```python
from build123d import *

# Parameters (mm, degrees)
F0_R           = 55
F1_DEPTH       = 8
F3_D           = 4
F4_D           = 3.75
F4_CBORE_D     = 6.75
F4_CBORE_DEPTH = 3
F5_W           = 80.514036
F5_H           = 245.416
F5_W_2         = 74.904691
F6_DEPTH       = 25


with BuildPart() as f1:
    # F0 (on Top) → F1 (new body)
    with BuildSketch(Plane.XY):
        with BuildLine():
            Line((105, 90), (105, 105))
            Line((105, 105), (90, 105))
            add(Edge.make_bspline(
                [(-90, 105), (-90, 62.5), (0, 62.5), (90, 62.5), (90, 105)],
                knots=[3.141593, 3.141593, 3.141593, 4.712389, 4.712389, 6.283185, 6.283185, 6.283185], degree=2, weights=[1, 0.707107, 1, 0.707107, 1]))
            Line((-90, 105), (-105, 105))
            Line((-105, 105), (-105, 90))
            add(Edge.make_bspline(
                [(-105, -90), (-62.5, -90), (-62.5, 0), (-62.5, 90), (-105, 90)],
                knots=[3.141593, 3.141593, 3.141593, 4.712389, 4.712389, 6.283185, 6.283185, 6.283185], degree=2, weights=[1, 0.707107, 1, 0.707107, 1]))
            Line((-105, -90), (-105, -105))
            Line((-105, -105), (-90, -105))
            add(Edge.make_bspline(
                [(90, -105), (90, -62.5), (0, -62.5), (-90, -62.5), (-90, -105)],
                knots=[0, 0, 0, 1.570796, 1.570796, 3.141593, 3.141593, 3.141593], degree=2, weights=[1, 0.707107, 1, 0.707107, 1]))
            Line((90, -105), (105, -105))
            Line((105, -105), (105, -90))
            add(Edge.make_bspline(
                [(105, 90), (62.5, 90), (62.5, 0), (62.5, -90), (105, -90)],
                knots=[0, 0, 0, 1.570796, 1.570796, 3.141593, 3.141593, 3.141593], degree=2, weights=[1, 0.707107, 1, 0.707107, 1]))
        make_face()
        Circle(F0_R, mode=Mode.SUBTRACT)
    extrude(amount=F1_DEPTH)

    # F3 (through all)
    with Locations(Plane.XY.offset(8)):
        with Locations((-100, 100), (100, 100), (100, -100), (-100, -100)):
            Hole(F3_D / 2)

    # F4 (through all)
    with Locations(Plane.XY.offset(8)):
        with Locations((-50, 50), (-50, -50), (50, -50), (50, 50)):
            CounterBoreHole(F4_D / 2, F4_CBORE_D / 2, F4_CBORE_DEPTH)

    # F5 (on Top) → F6 (cut)
    with BuildSketch(Plane.XY):
        Rectangle(F5_W, F5_H)
        with Locations((77.709363, 0)):
            Rectangle(F5_W_2, F5_H)
    extrude(amount=F6_DEPTH, mode=Mode.SUBTRACT)


solid = f1.part
```
Geometry check sheet. Reference: the model listing, model coordinates, mm. A direction names the side the tool comes from. Give positions to 0.01 mm unless a question says otherwise; leave off trailing zeros. Use one line per item in the form item = value.
Item 1: Scan lines: line 1 (Y direction, x = -50, z = 1.45) (3 decimals); line 2 (Y direction, x = -100, z = 3) (3 decimals); line 3 (Y direction, x = -75, z = 4.25). Record each from-to range of solid material in increasing order.
Results list:
line_1 = -69.662 to -51.875, -48.125 to -22.913, 22.913 to 48.125, 51.875 to 69.662
line_2 = -105 to -102, -98 to -89.375, 89.375 to 98, 102 to 105
line_3 = -81.51 to -63.75, 63.75 to 81.51
Item 2: Sectioned sample at A-A on x = -100. Count the separate pieces of the cut face and the enclosed holes in it, plus the area to 3 significant figures.
Results list:
separate_pieces = 4
enclosed_holes = 0
area = 186 mm2
Item 3: Mould release check, pull along X, two halves, no side actions. Record for faces 3 (the flat face through (-40.257, 52, 4)), 4 (the flat face through (-97, 105, 4)), 5 (the cylindrical face through (-51.01, 51.58, 2.46)): released by +X, released by -X, zero draft, split by the parting line, or undercut.
Results list:
face_3 = released by +X
face_4 = zero draft
face_5 = undercut
Item 4: Depth check by flat-ended pin: pin 1 Ø3 at (x, y) = (-100, -100) entering from -Z; pin 2 Ø2 at (x, z) = (-72, 5.5) entering from -Y. Enter the tip coordinate at first touch or a pass-through.
Results list:
pin_1 = through
pin_2 = -80.14
Item 5: Access from +Z, -Z, +X, -X, +Y, -Y to the whole of each face (thin tool, end or side, straight path). Record for faces 1 (the cylindrical face through (-101.075, -98.314, 3.944)), 2 (the flat face through (-48.5, -51.5, 5)).
Results list:
face_1 = +Z, -Z
face_2 = +Z
